Geometry: final body of the model. Coordinates: model frame, mm. A direction names the side the tool comes from. Coordinates: 2 decimals unless noted, no trailing zeros. Order: outer loops, then holes, each group sorted by start corner. A loop starts at its lowest first (then second) coordinate and runs counter-clockwise, first axis right, second up. Notation, with made-up numbers: (37.25, -6) -> (50.25, -6) arc R17 ccw to (50.25, 18) -> close; hole circle Ø5 at (-11, 26.5). An arc over 180 degrees is marked (long way). Use one line per item in the form item = value.
Autodesk Inventor part; units mm, degrees
ref_plane "YZ Plane" through (0, 0, 0) normal (1, 0, 0) x (0, 1, 0)
ref_plane "XZ Plane" through (0, 0, 0) normal (0, 1, 0) x (-1, 0, 0)
ref_plane "XY Plane" through (0, 0, 0) normal (0, 0, 1) x (1, 0, 0)
sketch "Sketch1" plane through (0, 0, 0) normal (0, 1, 0) x (-1, 0, 0)
  line L0 (25.4, 31.75) -> (-25.4, 31.75)
  line L1 (-25.4, 31.75) -> (-25.4, -31.75)
  line L2 (-25.4, -31.75) -> (25.4, -31.75)
  line L3 (25.4, -31.75) -> (25.4, 31.75)
  line L4 (25.4, 31.75) -> (-25.4, -31.75) construction
  line L5 (-25.4, 31.75) -> (25.4, -31.75) construction
  point P0 (0, 0)
  dimension "d0" = 50.8
  dimension "d1" = 63.5
extrude "Extrusion1" add sketch "Sketch1" along normal blind 5
sketch "Sketch2" plane through (0, 5, 0) normal (0, 1, 0) x (1, 0, 0)
  line L0 (25.4, 31.75) -> (-25.4, 31.75) construction
  line L1 (-25.4, -31.75) -> (25.4, -31.75) construction
  line L2 (-25.4, 31.75) -> (-25.4, -31.75) construction
  line L3 (-25.4, 0) -> (25.4, 0) construction
  line L4 (25.4, -31.75) -> (25.4, 31.75) construction
  line L5 (0, 31.75) -> (0, 0) construction
  line L6 (0, 0) -> (0, -31.75) construction
  line L7 (0, 15.875) -> (-25.4, 15.875) construction
  line L8 (-13.97, 15.875) -> (-11.43, 15.875) construction
  line L9 (-13.97, 13.275) -> (-11.43, 13.275)
  line L10 (-11.43, 18.475) -> (-13.97, 18.475)
  arc A0 (-13.97, 18.475) -> (-13.97, 13.275) centre (-13.97, 15.875) ccw
  arc A1 (-11.43, 13.275) -> (-11.43, 18.475) centre (-11.43, 15.875) ccw
  line L11 (0, 15.875) -> (25.4, 15.875) construction
  line L12 (13.97, 13.275) -> (11.43, 13.275)
  line L13 (11.43, 18.475) -> (13.97, 18.475)
  arc A2 (13.97, 13.275) -> (13.97, 18.475) centre (13.97, 15.875) ccw
  arc A3 (11.43, 18.475) -> (11.43, 13.275) centre (11.43, 15.875) ccw
  line L14 (-13.97, -13.275) -> (-11.43, -13.275)
  line L15 (-11.43, -18.475) -> (-13.97, -18.475)
  arc A4 (-13.97, -13.275) -> (-13.97, -18.475) centre (-13.97, -15.875) ccw
  arc A5 (-11.43, -18.475) -> (-11.43, -13.275) centre (-11.43, -15.875) ccw
  arc A6 (11.43, -13.275) -> (11.43, -18.475) centre (11.43, -15.875) ccw
  line L16 (13.97, -13.275) -> (11.43, -13.275)
  line L17 (11.43, -18.475) -> (13.97, -18.475)
  arc A7 (13.97, -18.475) -> (13.97, -13.275) centre (13.97, -15.875) ccw
  point P0 (-12.7, 15.875)
  point P1 (-12.7, 13.275)
  point P2 (-12.7, 18.475)
  dimension "d4" = 11.43
  dimension "d5" = 13.97
  dimension "d6" = 5.2
extrude "Extrusion2" cut sketch "Sketch2" against normal blind 5
sketch "Sketch3" plane through (25.4, 0, -31.75) normal (0, 0, -1) x (-1, 0, 0)
  line L0 (0, 0) -> (50.8, 0) construction
  line L1 (50.8, 0) -> (0, 0)
  line L2 (0, 0) -> (0, 31.75)
  line L3 (0, 31.75) -> (50.8, 31.75)
  line L4 (50.8, 31.75) -> (50.8, 0)
  point P0 (25.4, 0)
  dimension "d9" = 31.75
extrude "Extrusion3" add sketch "Sketch3" along normal blind 5
sketch "Sketch4" plane through (-25.4, 31.75, -31.75) normal (0, 1, 0) x (1, 0, 0)
  line L0 (0, 5) -> (50.8, 5) construction
  line L1 (50.8, -63.5) -> (50.8, 0) construction
  line L2 (0, 5) -> (50.8, 5)
  line L3 (50.8, 5) -> (50.8, -33.1)
  line L4 (50.8, -33.1) -> (0, -33.1)
  line L5 (0, -33.1) -> (0, 5)
  point P0 (25.4, -31.75)
  dimension "d12" = 38.1
extrude "Extrusion4" add sketch "Sketch4" along normal blind 5
sketch "Sketch5" plane through (-25.4, 36.75, -31.75) normal (0, 1, 0) x (1, 0, 0)
  line L0 (39.37, -50.225) -> (36.83, -50.225) construction
  arc A0 (36.83, -45.025) -> (36.83, -50.225) centre (36.83, -47.625) ccw construction
  line L1 (36.83, -45.025) -> (39.37, -45.025) construction
  arc A1 (39.37, -50.225) -> (39.37, -45.025) centre (39.37, -47.625) ccw construction
  arc A2 (36.83, -13.275) -> (36.83, -18.475) centre (36.83, -15.875) ccw
  line L2 (36.83, -13.275) -> (39.37, -13.275)
  arc A3 (39.37, -18.475) -> (39.37, -13.275) centre (39.37, -15.875) ccw
  line L3 (39.37, -18.475) -> (36.83, -18.475)
  arc A4 (11.43, -45.025) -> (11.43, -50.225) centre (11.43, -47.625) ccw construction
  line L4 (11.43, -45.025) -> (13.97, -45.025) construction
  arc A5 (13.97, -50.225) -> (13.97, -45.025) centre (13.97, -47.625) ccw construction
  line L5 (13.97, -50.225) -> (11.43, -50.225) construction
  line L6 (11.43, -13.275) -> (13.97, -13.275)
  arc A6 (13.97, -18.475) -> (13.97, -13.275) centre (13.97, -15.875) ccw
  line L7 (13.97, -18.475) -> (11.43, -18.475)
  arc A7 (11.43, -13.275) -> (11.43, -18.475) centre (11.43, -15.875) ccw
  line L8 (50.8, -63.5) -> (50.8, 0) construction
  line L9 (50.8, 0) -> (0, 0) construction
  line L10 (0, 0) -> (0, -63.5) construction
  line L11 (0, -63.5) -> (50.8, -63.5) construction
  point P0 (25.4, -31.75)
extrude "Extrusion5" cut sketch "Sketch5" against normal blind 5
properties part number "hanging_bracket_t-slot-2inx1in"
1) Pull-direction query (Y, two-part tool) for faces 3 (the flat face through (-13, 34, -13.275)), 4 (the flat face through (0, 19, -31.75)), 5 (the flat face through (0, 0, -2)); classes: released by +Y, released by -Y, zero draft, split by the parting line, or undercut.
Results found:
face_3 = zero draft
face_4 = undercut
face_5 = released by -Y
2) Access query for faces 1 (the flat face through (0, 18, -36.75)), 2 (the cylindrical face through (-16.57, 2.54, -15.93)). Directions: +Z, -Z, +X, -X, +Y, -Y. A direction counts if a zero-diameter tool reaches every point of the face in a straight line with its end or side. Return the directions, or none.
Results found:
face_1 = -Z, +X, -X, +Y, -Y
face_2 = +Y, -Y
3) Section A-A, the plane z = -4. Output: boundary loops of the cut face in (x, y).
Results found:
outline = (-25.4, 0) -> (25.4, 0) -> (25.4, 5) -> (-25.4, 5) -> close; (-25.4, 31.75) -> (25.4, 31.75) -> (25.4, 36.75) -> (-25.4, 36.75) -> close
4) Section C-C, the plane z = 16. Output: boundary loops of the cut face in (x, y).
Results found:
outline = (-25.4, 0) -> (-16.57, 0) -> (-16.57, 5) -> (-25.4, 5) -> close; (-8.83, 0) -> (8.83, 0) -> (8.83, 5) -> (-8.83, 5) -> close; (16.57, 0) -> (25.4, 0) -> (25.4, 5) -> (16.57, 5) -> close
5) Section D-D, the plane x = -2. Output: boundary loops of the cut face in (y, z).
Results found:
outline = (0, -36.75) -> (36.75, -36.75) -> (36.75, 1.35) -> (31.75, 1.35) -> (31.75, -31.75) -> (5, -31.75) -> (5, 31.75) -> (0, 31.75) -> close
6) Contact query for flat-ended pins moving along their axis: P1, Ø13.5, axis at x = -2.5, y = 18.5, coming from the +Z side; P2, Ø1.3, axis at x = 12.5, y = 35, coming from the +Z side; P3, Ø5, axis at x = -17.5, z = 20, coming from the +Y side. Output: stop coordinate, or through.
Results found:
P1 = -31.75
P2 = 1.35
P3 = 5
7) Section B-B, the plane x = 12.5. Output: boundary loops of the cut face in (y, z) (3 decimals).
Results found:
outline = (0, -36.75) -> (36.75, -36.75) -> (36.75, -18.475) -> (31.75, -18.475) -> (31.75, -31.75) -> (5, -31.75) -> (5, -18.475) -> (0, -18.475) -> close; (0, -13.275) -> (5, -13.275) -> (5, 13.275) -> (0, 13.275) -> close; (0, 18.475) -> (5, 18.475) -> (5, 31.75) -> (0, 31.75) -> close; (31.75, -13.275) -> (36.75, -13.275) -> (36.75, 1.35) -> (31.75, 1.35) -> close
8) Material intervals for probe 1 along Z at (x, y) = (11, 4); probe 2 along Y at (x, z) = (15, -22.5); probe 3 along Z at (x, y) = (3, 34.5), sorted ascending. Write a range as from..to.
Results found:
probe_1 = -36.75..-18.44, -13.31..13.31, 18.44..31.75
probe_2 = 0..5, 31.75..36.75
probe_3 = -36.75..1.35
